Model file for the job. Use its own axes, mm. Round coordinates to 2 decimals unless told otherwise and drop trailing zeros. Loops run counter-clockwise (first coordinate to the right, second up) from the corner with the lowest first, then second, coordinate; pieces in that order, holes last. Notation, with made-up numbers: M 67,28 L 108,28 A13 cw 108,45 Z; hole C 30,-7 d3. An arc over 180 degrees is marked long. Use a Markdown table: item, result. Add a question column.
Item 1: Saw through at D-D on y = 1.5. Give the number of separate pieces and of enclosed holes in the cut face, then the cut area to 3 significant figures.
Item 2: Wall check: L1, parallel to Z at x = 0, y = 4; L2, parallel to X at y = 0.3, z = 23.5; L3, parallel to X at y = 3.35, z = -30.25. Give the ranges that are in metal, low to high. Write a range as from..to.
Item 3: Saw through at A-A on z = 27.5. Write the cut outline in (x, y).
Item 4: Saw through at C-C on x = 44.5. Write the cut outline in (y, z).
Item 5: Saw through at B-B on z = 71. Write the cut outline in (x, y).
Item 6: Pin check, flat tips, straight feed: P1, Ø1, axis at y = 1, z = -67.5, coming from the -X side; P2, Ø2.5, axis at y = 1.5, z = 5.5, coming from the -X side. Stop position of each tip, or through.
```python
from build123d import *

# Parameters (mm, degrees)
SKETCH_1_W          = 80
SKETCH_1_H          = 180
EXTRUDE_1_DEPTH     = 5
HOLE_WIZARD_1_D     = 3.5
HOLE_WIZARD_2_D     = 4.5
HOLE_WIZARD_3_D     = 23
HOLE_WIZARD_4_D     = 9
SKETCH_13_W         = 30
SKETCH_13_H         = 70
EXTRUDE_2_DEPTH     = 5
EXTRUDE_3_DEPTH     = 5
HOLE_WIZARD_5_D     = 3.5
CUT_EXTRUDE_1_DEPTH = 5
HOLE_WIZARD_6_D     = 3.5
HOLE_WIZARD_7_D     = 3.5
HOLE_WIZARD_8_D     = 3.3
HOLE_WIZARD_9_D     = 3.5


with BuildPart() as part:
    # 草图1 → 凸台-拉伸1 (new body)
    with BuildSketch(Plane(origin=(0, 0, 0), x_dir=(1, 0, 0), z_dir=(0, 1, 0))):
        Rectangle(SKETCH_1_W, SKETCH_1_H)
    extrude(amount=EXTRUDE_1_DEPTH)

    # 孔1 (through all)
    with Locations(Plane(origin=(0, 5, 0), x_dir=(1, 0, 0), z_dir=(0, 1, 0))):
        with Locations((-31, 85.25), (-6, 85.25), (-6, 30.25), (-31, 30.25), (6, -8.45), (6, 46.55), (31, 46.55), (31, -8.45)):
            Hole(HOLE_WIZARD_1_D / 2)

    # 孔2 (through all)
    with Locations(Plane(origin=(0, 5, 0), x_dir=(1, 0, 0), z_dir=(0, 1, 0))):
        with Locations((0, -71), (25.11473671, -27.5), (-25.11473671, -27.5)):
            Hole(HOLE_WIZARD_2_D / 2)

    # 孔3 (through all)
    with Locations(Plane(origin=(0, 5, 0), x_dir=(1, 0, 0), z_dir=(0, 1, 0))):
        with Locations((0, -42)):
            Hole(HOLE_WIZARD_3_D / 2)

    # 孔4 (through all)
    with Locations(Plane(origin=(0, 5, 0), x_dir=(1, 0, 0), z_dir=(0, 1, 0))):
        with Locations((0, -61.25)):
            Hole(HOLE_WIZARD_4_D / 2)

    # 草图13 → 凸台-拉伸2 (add)
    with BuildSketch(Plane(origin=(0, 5, 0), x_dir=(1, 0, 0), z_dir=(0, 1, 0))):
        with Locations((-55, -55)):
            Rectangle(SKETCH_13_W, SKETCH_13_H)
        with Locations((55, -55)):
            Rectangle(SKETCH_13_W, SKETCH_13_H)
    extrude(amount=-EXTRUDE_2_DEPTH)

    # 草图15 → 凸台-拉伸3 (add)
    with BuildSketch(Plane(origin=(0, 5, 0), x_dir=(1, 0, 0), z_dir=(0, 1, 0))):
        Polygon((-40, 10), (-70, -20), (-61.514718626, -20), (-40, 1.514718626), align=None)
        Polygon((61.514718626, -20), (70, -20), (40, 10), (40, 1.514718626), align=None)
    extrude(amount=-EXTRUDE_3_DEPTH)

    # 孔5 (through all)
    with Locations(Plane(origin=(0, 5, 0), x_dir=(1, 0, 0), z_dir=(0, 1, 0))):
        with Locations((-66.5, -57), (66.5, -57)):
            Hole(HOLE_WIZARD_5_D / 2)

    # 草图19 → 切除-拉伸1 (cut)
    with BuildSketch(Plane(origin=(0, 5, 0), x_dir=(1, 0, 0), z_dir=(0, 1, 0))):
        Polygon((-70, -67), (-30.162831426, -90), (-70, -90), align=None)
        Polygon((30.162831426, -90), (70, -67), (70, -90), align=None)
    extrude(amount=-CUT_EXTRUDE_1_DEPTH, mode=Mode.SUBTRACT)

    # 孔6 (through all)
    with Locations(Plane(origin=(0, 5, 0), x_dir=(1, 0, 0), z_dir=(0, 1, 0))):
        with Locations((-66.5, -23.5), (66.5, -23.5)):
            Hole(HOLE_WIZARD_6_D / 2)

    # 孔7 (through all)
    with Locations(Plane(origin=(0, 5, 0), x_dir=(1, 0, 0), z_dir=(0, 1, 0))):
        with Locations((49.5, -36.5)):
            Hole(HOLE_WIZARD_7_D / 2)

    # 孔8 (through all)
    with Locations(Plane(origin=(0, 5, 0), x_dir=(1, 0, 0), z_dir=(0, 1, 0))):
        with Locations((-12.784, -5), (16.216, 82.5)):
            Hole(HOLE_WIZARD_8_D / 2)

    # 孔9 (through all)
    with Locations(Plane(origin=(0, 5, 0), x_dir=(1, 0, 0), z_dir=(0, 1, 0))):
        with Locations((-66.5, -36.5)):
            Hole(HOLE_WIZARD_9_D / 2)


solid = part.part
```
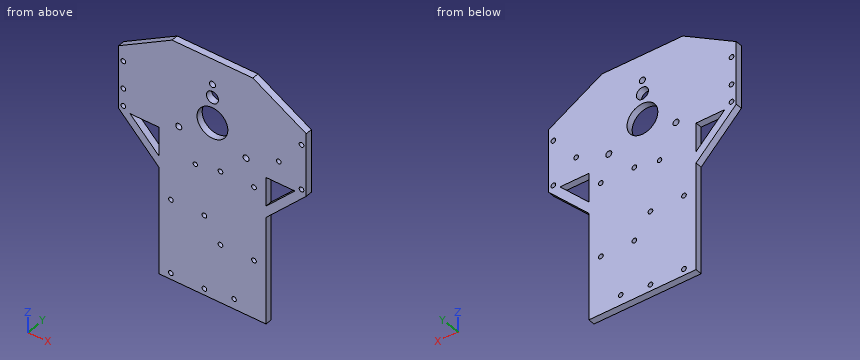
Entries:
| question | item | result |
|---|---|---|
| 1 | separate pieces | 1 |
| 1 | enclosed holes | 23 |
| 1 | area | 17,400 mm2 |
| 2 | L1 | -90..30.5, 53.5..56.75, 65.75..68.75, 73.25..90 |
| 2 | L2 | -70..-68.25, -64.75..64.75, 68.25..70 |
| 2 | L3 | -40..-32.75, -29.25..-7.75, -4.25..40 |
| 3 | outline | M -70,0 L -27.36,0 L -27.36,5 L -70,5 Z; M -22.86,0 L 22.86,0 L 22.86,5 L -22.86,5 Z; M 27.36,0 L 70,0 L 70,5 L 27.36,5 Z |
| 4 | outline | M 0,-5.5 L 5,-5.5 L 5,2.99 L 0,2.99 Z; M 0,20 L 5,20 L 5,81.72 L 0,81.72 Z |
| 5 | outline | M -63.07,0 L -2.25,0 L -2.25,5 L -63.07,5 Z; M 2.25,0 L 63.07,0 L 63.07,5 L 2.25,5 Z |
| 6 | P1 | x = -40 |
| 6 | P2 | x = -56.75 |
